The listing builds one solid part. Answer for the finished solid, in the listing's coordinates (mm). A direction names the side the tool comes from. Round coordinates to 2 decimals unless told otherwise and drop trailing zeros. Write each loop counter-clockwise with the first axis right and the second up, starting at its lowest first coordinate (ties: lowest second). Pieces come first, ordered by that corner, then holes. Notation, with made-up numbers: (7.5, 35.5) - (12.5, 35.5) arc R26 ccw to (12.5, 58.5) - close; hole circle Ø2 at (56, 86.25). An arc over 180 degrees is marked (long way). Answer as CSV lines item,"result". Start each with the question number.
Item 1: A cutting plane is placed at C-C on x = 10.5. Determine the outline of the cut face in (y, z), and give its area (3 significant figures).
Item 2: A cutting plane is placed at D-D on z = 10.5. Determine the outline of the cut face in (x, y).
Item 3: Straight lines are drawn through the part: line 1 along X through (y, z) = (71.5, 5.5); line 2 along X through (y, z) = (38.25, 1.5); line 3 along Y through (x, z) = (36.5, 2.15). For each, find the intervals that lie inside material, in ascending order. Write a range as [from, to].
Item 4: A cutting plane is placed at B-B on y = 38.25. Determine the outline of the cut face in (x, z).
Item 5: A cutting plane is placed at A-A on z = 1.75. State how many separate pieces and enclosed holes the cut face has, and give its area (3 significant figures).
Item 6: For a pull along Z with two mould halves and no side action, classify faces 6 (the flat face through (16.5, 65, 7)), 7 (the flat face through (21, 75, 14.5)), 8 (the flat face through (7.8, 38.4, 6)), 9 (the flat face through (22.758, 1.479, 13.778)) as pulls with the +Z half, pulls with the -Z half, needs draft (parallel to the pull), parting line crosses it, or undercut.
Item 7: Which of the six approach directions +Z, -Z, +X, -X, +Y, -Y give full straight-line access (tool end or side, diameter ignored) to faces 1 (the flat face through (13.5, 10, 9)), 2 (the cylindrical face through (10.13, 0.39, 1.52)), 3 (the flat face through (25.5, 12, 7)), 4 (the cylindrical face through (20.9, 75, 9.5)), 5 (the flat face through (4, 39, 3))?
Item 8: Flat-ended cylindrical pins translate along their axes: pin 1 (6.5 mm diameter, centred on x = 5.5, y = 53.75, fed in from +Z); pin 2 (4 mm diameter, centred on x = 13.5, z = 10.5, fed in from -Y); pin 3 (0.5 mm diameter, centred on y = 77, z = 17, fed in from -X). Find the tip coordinate at first contact, or state that the pin passes through.
```python
from build123d import *

# Parameters (mm, degrees)
SKETCH_W        = 42
SKETCH_H        = 76.5
SKETCH_R        = 13
SKETCH_R_2      = 2
PAD_DEPTH       = 3
PAD001_DEPTH    = 3
POCKET_DEPTH    = 3
PAD002_DEPTH    = 12
SKETCH004_W     = 5.5
SKETCH004_H     = 2.5
SKETCH004_H_2   = 8.5
PAD003_DEPTH    = 1
SKETCH005_W     = 5.5
SKETCH005_H     = 2.5
SKETCH005_H_2   = 8.5
PAD004_DEPTH    = 1
POCKET001_DEPTH = 77.501
CHAMFER_SIZE    = 11
CHAMFER001_SIZE = 10
FILLET_R        = 5
CHAMFER002_SIZE = 0.9


with BuildPart() as part:
    # Sketch → Pad (new body)
    with BuildSketch(Plane.XY):
        with Locations((21, 38.25)):
            Rectangle(SKETCH_W, SKETCH_H)
        with Locations((21, 38.25)):
            Circle(SKETCH_R, mode=Mode.SUBTRACT)
        with Locations((5.5, 22.75)):
            Circle(SKETCH_R_2, mode=Mode.SUBTRACT)
        with Locations((5.5, 53.75)):
            Circle(SKETCH_R_2, mode=Mode.SUBTRACT)
        with Locations((36.5, 53.75)):
            Circle(SKETCH_R_2, mode=Mode.SUBTRACT)
        with Locations((36.5, 22.75)):
            Circle(SKETCH_R_2, mode=Mode.SUBTRACT)
    extrude(amount=PAD_DEPTH)

    # Sketch001 → Pad001 (new body)
    with BuildSketch(Plane.XY.offset(3)):
        with BuildLine():
            Line((13.5, 76.5), (28.5, 76.5))
            Line((28.5, 76.5), (28.5, 52.383294))
            ThreePointArc((28.5, 24.116706), (37, 38.25), (28.5, 52.383294))
            Line((28.5, 0), (28.5, 24.116706))
            Line((13.5, 0), (28.5, 0))
            Line((13.5, 24.116706), (13.5, 0))
            ThreePointArc((13.5, 52.383294), (5, 38.25), (13.5, 24.116706))
            Line((13.5, 52.383294), (13.5, 76.5))
        make_face()
    extrude(amount=PAD001_DEPTH)

    # Sketch003 → Pocket (cut)
    with BuildSketch(Plane.XY.offset(6)):
        with BuildLine():
            Line((25.5, 50.446311), (25.5, 73.5))
            Line((25.5, 73.5), (16.5, 73.5))
            Line((16.5, 73.5), (16.5, 50.446311))
            ThreePointArc((16.5, 50.446311), (8, 38.25), (16.5, 26.053689))
            Line((16.5, 3), (16.5, 26.053689))
            Line((25.5, 3), (16.5, 3))
            Line((25.5, 26.053689), (25.5, 3))
            ThreePointArc((25.5, 26.053689), (34, 38.25), (25.5, 50.446311))
        make_face()
    extrude(amount=-POCKET_DEPTH, mode=Mode.SUBTRACT)

    # Sketch007 → Pad002 (new body)
    with BuildSketch(Plane.XY.offset(6)):
        Polygon((13.5, 76.5), (28.5, 76.5), (28.5, 61.5), (25.5, 61.5), (25.5, 73.5), (16.5, 73.5), (16.5, 61.5), (13.5, 61.5), align=None)
        Polygon((28.5, 0), (28.5, 15), (25.5, 15), (25.5, 3), (16.5, 3), (16.5, 15), (13.5, 15), (13.5, 0), align=None)
    extrude(amount=PAD002_DEPTH)

    # Sketch004 → Pad003 (new body)
    with BuildSketch(Plane.XZ):
        with Locations((21, 16.75)):
            Rectangle(SKETCH004_W, SKETCH004_H)
        with Locations((21, 4.25)):
            Rectangle(SKETCH004_W, SKETCH004_H_2)
    extrude(amount=PAD003_DEPTH)

    # Sketch005 → Pad004 (new body)
    with BuildSketch(Plane(origin=(0, 76.5, 0), x_dir=(-1, 0, 0), z_dir=(0, 1, 0))):
        with Locations((-21, 16.75)):
            Rectangle(SKETCH005_W, SKETCH005_H)
        with Locations((-21, 4.25)):
            Rectangle(SKETCH005_W, SKETCH005_H_2)
    extrude(amount=PAD004_DEPTH)

    # Sketch006 → Pocket001 (cut, through all)
    with BuildSketch(Plane.XZ):
        with BuildLine():
            ThreePointArc((18.5, 12), (21, 9.5), (23.5, 12))
            Line((23.5, 13.035534), (23.5, 12))
            Line((22.035534, 14.5), (23.5, 13.035534))
            Line((19.964466, 14.5), (22.035534, 14.5))
            Line((18.5, 13.035534), (19.964466, 14.5))
            Line((18.5, 12), (18.5, 13.035534))
        make_face()
    extrude(amount=-POCKET001_DEPTH, mode=Mode.SUBTRACT)

    # Chamfer
    chamfer_edges = [part.edges().sort_by_distance(p)[0] for p in [
        (15, 61.5, 18),
        (27, 61.5, 18),
        (27, 15, 18),
        (15, 15, 18),
    ]]
    chamfer(chamfer_edges, length=CHAMFER_SIZE)

    # Chamfer001
    chamfer001_edges = [part.edges().sort_by_distance(p)[0] for p in [
        (0, 0, 1.5),
        (42, 0, 1.5),
        (0, 76.5, 1.5),
        (42, 76.5, 1.5),
    ]]
    chamfer(chamfer001_edges, length=CHAMFER001_SIZE)

    # Fillet
    fillet_edges = [part.edges().sort_by_distance(p)[0] for p in [
        (10, 76.5, 1.5),
        (0, 66.5, 1.5),
        (0, 10, 1.5),
        (10, 0, 1.5),
        (32, 0, 1.5),
        (42, 10, 1.5),
        (32, 76.5, 1.5),
        (42, 66.5, 1.5),
    ]]
    fillet(fillet_edges, radius=FILLET_R)

    # Chamfer002
    chamfer002_edges = [part.edges().sort_by_distance(p)[0] for p in [
        (21, 77.5, 15.5),
        (21, -1, 15.5),
    ]]
    chamfer(chamfer002_edges, length=CHAMFER002_SIZE)


solid = part.part
```
Geometry says:
1,outline,"(0.25, 0) - (30.59, 0) - (30.59, 6) - (26.18, 6) - (26.18, 3) - (0.25, 3) - close; (45.91, 0) - (76.25, 0) - (76.25, 3) - (50.32, 3) - (50.32, 6) - (45.91, 6) - close"
1,area,"208 mm^2"
2,outline,"(13.5, 0) - (19, 0) - (19, 3) - (16.5, 3) - (16.5, 11.5) - (13.5, 11.5) - close; (13.5, 65) - (16.5, 65) - (16.5, 73.5) - (19, 73.5) - (19, 76.5) - (13.5, 76.5) - close; (23, 0) - (28.5, 0) - (28.5, 11.5) - (25.5, 11.5) - (25.5, 3) - (23, 3) - close; (23, 73.5) - (25.5, 73.5) - (25.5, 65) - (28.5, 65) - (28.5, 76.5) - (23, 76.5) - close"
3,line 1,"x = [13.5, 16.5], [25.5, 28.5]"
3,line 2,"x = [0, 8], [34, 42]"
3,line 3,"y = [4.5, 20.75], [24.75, 51.75], [55.75, 72]"
4,outline,"(0, 0) - (8, 0) - (8, 6) - (5, 6) - (5, 3) - (0, 3) - close; (34, 0) - (42, 0) - (42, 3) - (37, 3) - (37, 6) - (34, 6) - close"
5,separate pieces,"1"
5,enclosed holes,"5"
5,area,"2,440 mm^2"
6,face 6,"needs draft"
6,face 7,"undercut"
6,face 8,"pulls with the +Z half"
6,face 9,"undercut"
7,face 1,"+Z, -X, -Y"
7,face 2,"+Z, -Z, -X, -Y"
7,face 3,"+Z"
7,face 4,"+Y, -Y"
7,face 5,"+Z, -X"
8,pin 1,"stops at z = 3"
8,pin 2,"stops at y = 0"
8,pin 3,"stops at x = 18.25"
